```python
from build123d import *

# Parameters (mm, degrees)
SKETCH2_OUTSIDE_W   = 30.882
SKETCH2_OUTSIDE_H   = 30.882
SKETCH2_OUTSIDE_W_2 = 11
SKETCH2_OUTSIDE_H_2 = 14
CUT_EXTRUDE1_DEPTH  = 10.342159


with BuildPart() as part:
    # Sketch1 → Body Revolve (revolve)
    with BuildSketch(Plane.XY):
        with BuildLine():
            Line((-14.5, 7), (-17.5, 7))
            Line((-17.5, 7), (-17.5, 5))
            Line((-17.5, 5), (-21.095854812, 5))
            Line((-21.095854812, 5), (-21.5, 4.3))
            Line((-21.5, 4.3), (-21.904145188, 5))
            Line((-21.904145188, 5), (-41.8, 5))
            Line((-41.8, 5), (-42.5, 4.3))
            Line((-42.5, 4.3), (-42.5, 0))
            Line((-42.5, 0), (8.75, 0))
            ThreePointArc((8.75, 0), (2.639260414, 8.342469926), (-7.15784102, 5.032674431))
            Line((-7.15784102, 5.032674431), (-14.5, 7))
        make_face()
    revolve(axis=Axis((-9.81300365, 0, 0), (1, 0, 0)))

    # Sketch2 outside → Cut-Extrude1 (cut)
    with BuildSketch(Plane.ZY.offset(17.5)):
        Rectangle(SKETCH2_OUTSIDE_W, SKETCH2_OUTSIDE_H)
        Rectangle(SKETCH2_OUTSIDE_W_2, SKETCH2_OUTSIDE_H_2, mode=Mode.SUBTRACT)
    extrude(amount=-CUT_EXTRUDE1_DEPTH, mode=Mode.SUBTRACT)


solid = part.part
```
Input: part model. Units: mm. Frame: model coordinates. A direction names the side the tool comes from. Round coordinates to 2 decimals unless told otherwise and drop trailing zeros. Loops run counter-clockwise (first coordinate to the right, second up) from the corner with the lowest first, then second, coordinate; pieces in that order, holes last. Notation, with made-up numbers: (46.25, -18.5) -> (79.25, -18.5) arc R4 ccw to (79.25, -14.5) -> close; hole circle Ø7 at (-38, 87.25). An arc over 180 degrees is marked (long way). Use one line per item in the form item = value. Start each with the question number.
Item 1: Section query C-C on y = 0. Return the cut outline in (x, z), then the cut area to 3 significant figures.
Item 2: Contact query for flat-ended pins moving along their axis: pin 1 Ø8 at (x, z) = (-37.5, -1) entering from -Y; pin 2 Ø1 at (y, z) = (-7, -2.5) entering from +X; pin 3 Ø2 at (y, z) = (5.5, 1) entering from -X; pin 4 Ø10 at (y, z) = (-4, 3) entering from -X. Output: stop coordinate, or through.
Item 3: Material intervals for L1, parallel to X at y = 3.5, z = -3.5; L2, parallel to Y at x = 4, z = 3.75; L3, parallel to X at y = 0, z = 5.75, sorted ascending. Write a range as from..to.
Item 4: Section query A-A on z = 0. Return the cut outline in (x, y).
Item 5: Section query D-D on z = -7. Return the cut outline in (x, y), then the cut area to 3 significant figures.
Item 6: Set-up query: faces 4 (the face through (-19.32, -1.08, -4.88)), 5 (the face through (-16, -7, 0)), 6 (the face through (-16, 7, 0)), 7 (the face through (-14, 0, -5.5)), 8 (the face through (-14, 0, 5.5)). Return all of +Z, -Z, +X, -X, +Y, -Y with unobstructed straight access to the full face (end or side cutting, diameter ignored); none if empty.
Item 7: Section query B-B on x = -37. Return the cut outline in (y, z), then the cut area to 3 significant figures.
Item 8: Mould query, pull axis X, two halves, no side actions, for faces 1 (the face through (-17.5, -2, -5)), 2 (the face through (-9.25, -4.12, 3.78)), 3 (the face through (-31.99, -1.08, -4.88)). Classes: pulls with the +X half, pulls with the -X half, needs draft (parallel to the pull), parting line crosses it, or undercut.
Ans:
q1.outline = (-42.5, -4.3) -> (-41.8, -5) -> (-21.9, -5) -> (-21.5, -4.3) -> (-21.1, -5) -> (-17.5, -5) -> (-17.5, -5.5) -> (-8.9, -5.5) -> (-7.16, -5.03) arc R8.75 ccw (long way) to (-7.16, 5.03) -> (-8.9, 5.5) -> (-17.5, 5.5) -> (-17.5, 5) -> (-21.1, 5) -> (-21.5, 4.3) -> (-21.9, 5) -> (-41.8, 5) -> (-42.5, 4.3) -> close
q1.area = 592 mm^2
q2.pin_1 = -5
q2.pin_2 = 5.34
q2.pin_3 = -42.21
q2.pin_4 = -42.5
q3.L1 = -41.85..-21.88, -21.12..7.22
q3.L2 = -6.82..6.82
q3.L3 = -6.6..6.6
q4.outline = (-42.5, -4.3) -> (-41.8, -5) -> (-21.9, -5) -> (-21.5, -4.3) -> (-21.1, -5) -> (-17.5, -5) -> (-17.5, -7) -> (-14.5, -7) -> (-7.16, -5.03) arc R8.75 ccw (long way) to (-7.16, 5.03) -> (-14.5, 7) -> (-17.5, 7) -> (-17.5, 5) -> (-21.1, 5) -> (-21.5, 4.3) -> (-21.9, 5) -> (-41.8, 5) -> (-42.5, 4.3) -> close
q5.outline = circle Ø10.5 at (0, 0)
q5.area = 86.6 mm^2
q6.face_4 = -X
q6.face_5 = -X, -Y
q6.face_6 = -X, +Y
q6.face_7 = -Z, -X, +Y, -Y
q6.face_8 = +Z, -X, +Y, -Y
q7.outline = circle Ø10 at (0, 0)
q7.area = 78.5 mm^2
q8.face_1 = pulls with the -X half
q8.face_2 = undercut
q8.face_3 = needs draft
